Geometry: final body of the model. Coordinates: model frame, mm. A direction names the side the tool comes from. Give positions to 0.01 mm unless a question says otherwise; leave off trailing zeros. Loops run counter-clockwise (first coordinate to the right, second up) from the corner with the lowest first, then second, coordinate; pieces in that order, holes last. Notation, with made-up numbers: (0.25, 11) - (5.25, 11) arc R18 ccw to (5.25, 28) - close; hole circle Ø7 at (47.25, 25.25). An arc over 180 degrees is marked (long way). Answer in a Markdown table with one row per item.
Autodesk Fusion 360 part; units mm, degrees
sketch "Sketch1" plane through (0, 0, 0) normal (0, 0, 1) x (1, 0, 0)
  circle A0 centre (0, 0) radius 74
  circle A1 centre (0, 18) radius 25.5
  circle A2 centre (0, 0) radius 70
  circle A3 centre (0, 18) radius 29
  dimension "d1" = 148
  dimension "d2" = 51
  dimension "d3" = 18
  dimension "d4" = 140
  dimension "d5" = 58
extrude "Extrude1" add sketch "Sketch1" along normal blind 5 contours A0 | A2 | A3
extrude "Extrude2" add sketch "Sketch1" along normal blind 20
fillet "Fillet1" radius 10 2 edges at (-27.0375, 28.4868, 5) (-65.2629, -25.3131, 5)
Q1. Cut plane B-B (z = 7). Output: boundary loops of the cut face in (x, y), and give its area (3 significant figures).
Check values:
| item | result |
|---|---|
| outline | circle Ø148 at (0, 0); circle Ø66 at (0, 18); hole circle Ø132 at (0, 0); hole circle Ø51 at (0, 18) |
| area | 4,900 mm² |
Q2. Draft query along X for faces 3 (the flat face through (-1, -15, 0)), 4 (the cylindrical face through (-16.04, 72.24, 9.86)), 5 (the cylindrical face through (-5.5, 42.9, 9.9)). Return one class per face: pulls with the +X half, pulls with the -X half, needs draft (parallel to the pull), parting line crosses it, or undercut.
Check values:
| item | result |
|---|---|
| face 3 | needs draft |
| face 4 | parting line crosses it |
| face 5 | undercut |
Q3. Cut plane A-A (x = 0). Output: boundary loops of the cut face in (y, z), and give its area (3 significant figures).
Check values:
| item | result |
|---|---|
| outline | (-74, 0) - (-7.5, 0) - (-7.5, 20) - (-11, 20) - (-11, 15) arc R10 cw to (-21, 5) - (-60, 5) arc R10 cw to (-70, 15) - (-70, 20) - (-74, 20) - close; (43.5, 0) - (74, 0) - (74, 20) - (70, 20) - (70, 15) arc R10 cw to (60, 5) - (57, 5) arc R10 cw to (47, 15) - (47, 20) - (43.5, 20) - close |
| area | 796 mm² |
Q4. Material intervals for line 1 along Y through (x, z) = (0, 14.5); line 2 along Y through (x, z) = (19, 14.75); line 3 along X through (y, z) = (30, 15.5), sorted ascending.
Check values:
| item | result |
|---|---|
| line 1 | -74 to -69.99, -11.01 to -7.5, 43.5 to 47.01, 69.99 to 74 |
| line 2 | -71.52 to -67.37, -3.91 to 0.99, 35.01 to 39.91, 67.37 to 71.52 |
| line 3 | -67.65 to -63.25, -26.4 to -22.5, 22.5 to 26.4, 63.25 to 67.65 |
Q5. First-contact query: pin 1 (5 mm diameter, centred on x = 43, z = 4.5, fed in from +Y); pin 2 (1.5 mm diameter, centred on x = -31.5, z = 9.5, fed in from +Y); pin 3 (5 mm diameter, centred on x = -15, z = 16.5, fed in from -Y). Flat tips, straight axial feed; report the tip coordinate or a pass-through.
Check values:
| item | result |
|---|---|
| pin 1 | y = 61.93 |
| pin 2 | y = 67.31 |
| pin 3 | y = -72.94 |
Q6. Reachability of faces 1 (the flat face through (0, -8, 20)), 2 (the cylindrical face through (13.38, 43.73, 17.46)) from +Z, -Z, +X, -X, +Y, -Y: full face, straight path, thin tool, end or side. Return the list, or none.
Check values:
| item | result |
|---|---|
| face 1 | +Z, +X, -X, +Y, -Y |
| face 2 | +Z |
